Source: CAD feature listing. Evaluate the final solid. Frame: model axes, mm. Face numbers are marked on the shaded views. Give positions to 0.01 mm unless a question says otherwise; leave off trailing zeros. Write each loop counter-clockwise with the first axis right and the second up, starting at its lowest first coordinate (ties: lowest second). Pieces come first, ordered by that corner, then holes. Notation, with made-up numbers: (39, -12) -> (95, -12) arc R22 ccw to (95, 2) -> close; hole circle Ø2 at (75, 68). An arc over 180 degrees is marked (long way). Answer as a JSON object with one key per item and string values. Group by question number.
Item 1: Section query D-D on z = 15. Return the cut outline in (x, y), plus the area to 3 significant figures.
Item 2: Section query C-C on x = 90. Return the cut outline in (y, z).
Item 3: First-contact query: pin 1 Ø3 at (y, z) = (-22, -2) entering from -X (3 decimals); pin 2 Ø8 at (y, z) = (-6.5, 10.5) entering from +X; pin 3 Ø4 at (y, z) = (-16, -9.5) entering from -X. Flat tips, straight axial feed; report the tip coordinate or a pass-through.
Item 4: Ray query, probe 1 along Z at (x, y) = (0, -13.5); probe 2 along X at (y, z) = (-8.75, -8.5); probe 3 along Z at (x, y) = (90, -15.5). Return the intervals inside material, ascending. Write a range as from..to.
Item 5: Section query B-B on y = -8.25. Return the cut outline in (x, z), plus the area to 3 significant figures.
Item 6: Pull-direction query (Z, two-part tool) for the marked faces 1, 2 and 3; classes: pulls with the +Z half, pulls with the -Z half, needs draft (parallel to the pull), parting line crosses it, or undercut.
Item 7: Section query A-A on z = 0. Return the cut outline in (x, y).
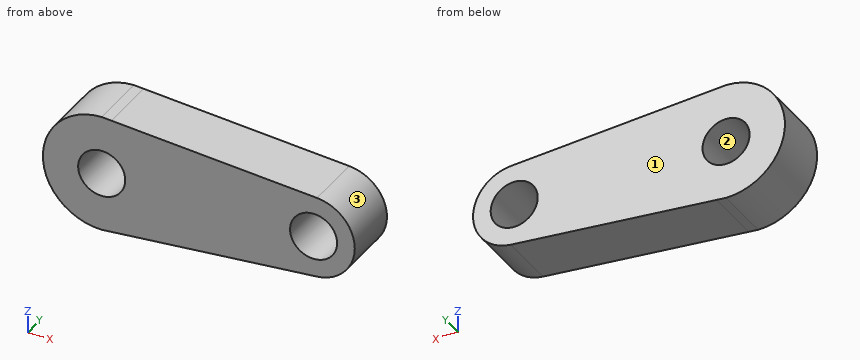
from build123d import *

# Parameters (mm, degrees)
F0_R     = 10
F1_DEPTH = 25


with BuildPart() as f1:
    # F0 (on Front) → F1 (new body)
    with BuildSketch(Plane.XZ):
        with BuildLine():
            Line((4.1054428346, 24.6606029758), (0, 25))
            ThreePointArc((0, 25), (-25, 0), (0, -25))
            Line((0, -25), (4.1054428346, -24.6606029758))
            ThreePointArc((4.1054428346, -24.6606029758), (19.0740146648, -16.1611251022), (25, 0))
            ThreePointArc((25, 0), (19.0740146648, 16.1611251022), (4.1054428346, 24.6606029758))
        make_face()
        Circle(F0_R, mode=Mode.SUBTRACT)
        with BuildLine():
            Line((91.4418067738, 17.4405043857), (4.1054428346, 24.6606029758))
            ThreePointArc((4.1054428346, 24.6606029758), (19.0740146648, 16.1611251022), (25, 0))
            ThreePointArc((25, 0), (19.0740146648, -16.1611251022), (4.1054428346, -24.6606029758))
            Line((4.1054428346, -24.6606029758), (91.4418067738, -17.4405043857))
            ThreePointArc((91.4418067738, -17.4405043857), (72.5, 0), (91.4418067738, 17.4405043857))
        make_face()
        with BuildLine():
            ThreePointArc((107.5, 0), (102.8740362463, 11.8536572723), (91.4418067738, 17.4405043857))
            ThreePointArc((91.4418067738, 17.4405043857), (72.5, 0), (91.4418067738, -17.4405043857))
            ThreePointArc((91.4418067738, -17.4405043857), (102.8740362463, -11.8536572723), (107.5, 0))
        make_face()
        with Locations((90, 0)):
            Circle(F0_R, mode=Mode.SUBTRACT)
    extrude(amount=F1_DEPTH)


solid = f1.part
Worked answers:
{
 "1": {"outline": "(-20, -25) -> (99.01, -25) -> (99.01, 0) -> (-20, 0) -> close", "area": "2,980 mm^2"},
 "2": {"outline": "(-25, -17.56) -> (0, -17.56) -> (0, -10) -> (-25, -10) -> close; (-25, 10) -> (0, 10) -> (0, 17.56) -> (-25, 17.56) -> close"},
 "3": {"pin 1": "x = -24.995", "pin 2": "x = 106.25", "pin 3": "x = -23.85"},
 "4": {"probe 1": "-25..-10, 10..25", "probe 2": "-23.51..-5.27, 5.27..84.73, 95.27..105.3", "probe 3": "-17.56..-10, 10..17.56"},
 "5": {"outline": "(0, -25) -> (91.44, -17.44) arc R17.5 ccw to (91.44, 17.44) -> (0, 25) arc R25 ccw to start; hole circle Ø20 at (0, 0); hole circle Ø20 at (90, 0)", "area": "4,660 mm^2"},
 "6": {"face 1": "needs draft", "face 2": "undercut", "face 3": "parting line crosses it"},
 "7": {"outline": "(-25, -25) -> (-10, -25) -> (-10, 0) -> (-25, 0) -> close; (10, -25) -> (80, -25) -> (80, 0) -> (10, 0) -> close; (100, -25) -> (107.5, -25) -> (107.5, 0) -> (100, 0) -> close"}
}
